Read the model definition and answer for the solid it produces. Units are mm, in the model's axes. Round coordinates to 2 decimals unless told otherwise and drop trailing zeros. Order: outer loops, then holes, each group sorted by start corner. A loop starts at its lowest first (then second) coordinate and runs counter-clockwise, first axis right, second up. Notation, with made-up numbers: (17, 48) - (55, 48) arc R23 cw to (55, 78) - close; hole circle Ø8 at (85, -7). An arc over 180 degrees is marked (long way). Answer as a JSON object with one key per item and string values. Group by question number.
Q1. A cutting plane is placed at C-C on x = -38. Determine the outline of the cut face in (y, z), and give its area (3 significant figures).
Q2. A cutting plane is placed at B-B on z = 0. Determine the outline of the cut face in (x, y).
Q3. A cutting plane is placed at D-D on y = -64.5. Determine the outline of the cut face in (x, z), and give its area (3 significant figures).
Q4. Given pin 1 Ø1 at (x, z) = (-33, 1) entering from +Y; pin 2 Ø2 at (y, z) = (-109.5, 0.5) entering from -X; pin 3 Ø1.2 at (y, z) = (-50.5, 0) entering from -X, each flat-ended and moving along its own axis, determine where each tip first touches the part or whether it passes through.
Q5. Consider line 1 (Z direction, x = -4, y = -113.5); line 2 (X direction, y = 2, z = 0.2); line 3 (X direction, y = -63.5, z = 1). Determine where each line is inside the solid, lowest interval first.
Q6. A cutting plane is placed at A-A on y = -10. Determine the outline of the cut face in (x, z), and give its area (3 significant figures).
```python
from build123d import *

# Parameters (mm, degrees)
PAD_DEPTH    = 2.4
POCKET_DEPTH = 1.2
CHAMFER_SIZE = 1


with BuildPart() as part:
    # Sketch001 → Pad (new body, symmetric)
    with BuildSketch(Plane.XY):
        with BuildLine():
            ThreePointArc((-35.969784, -57.54415), (-33.691358, -77.55321), (-29.473826, -97.244988))
            ThreePointArc((-29.473826, -97.244988), (-17.916413, -119.460908), (2, -134.64173))
            Line((2, -134.64173), (2, 84.534861))
            Line((-45.930419, 96.485256), (2, 84.534861))
            Line((-35.969784, -57.54415), (-45.930419, 96.485256))
        make_face()
    extrude(amount=PAD_DEPTH, both=True)

    # Sketch → Pocket (cut, symmetric)
    with BuildSketch(Plane.XY):
        with BuildLine():
            Line((0, 85.033517), (0, -130.966483))
            ThreePointArc((-27.154362, -96.628473), (-17.140793, -116.615568), (0, -130.966483))
            ThreePointArc((-33.574786, -57.389272), (-31.322854, -77.165669), (-27.154362, -96.628473))
            Line((-33.574786, -57.389272), (-43.485993, 95.875793))
            Line((-43.485993, 95.875793), (0, 85.033517))
        make_face()
    extrude(amount=POCKET_DEPTH, both=True, mode=Mode.SUBTRACT)

    # Chamfer
    chamfer_edges = [part.edges().sort_by_distance(p)[0] for p in [
        (2, -134.64173, 0),
    ]]
    chamfer(chamfer_edges, length=CHAMFER_SIZE)


solid = part.part
```
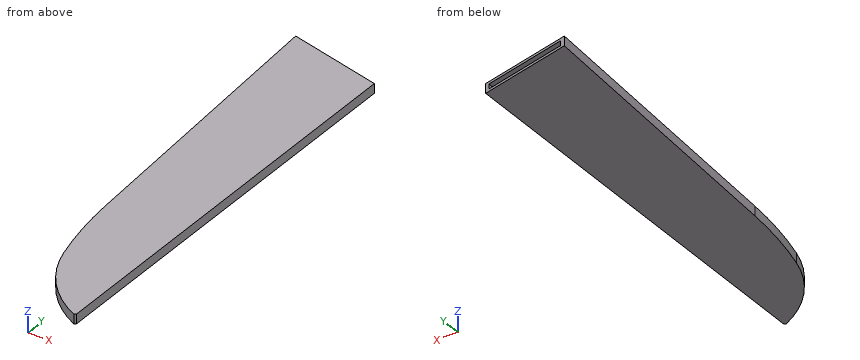
Result set:
{
 "1": {"outline": "(-26.15, -2.4) - (94.51, -2.4) - (94.51, -1.2) - (11.04, -1.2) - (11.04, 1.2) - (94.51, 1.2) - (94.51, 2.4) - (-26.15, 2.4) - close", "area": "379 mm²"},
 "2": {"outline": "(-45.93, 96.49) - (-35.97, -57.54) arc R206.4 ccw to (-29.47, -97.24) arc R57.4 ccw to (1.1, -134.22) - (2, -133.64) - (2, 84.53) - (0, 85.03) - (0, -130.97) arc R55 cw to (-27.15, -96.63) arc R204 cw to (-33.57, -57.39) - (-43.49, 95.88) - close"},
 "3": {"outline": "(-35.4, -2.4) - (2, -2.4) - (2, 2.4) - (-35.4, 2.4) - close; hole (-32.99, -1.2) - (0, -1.2) - (0, 1.2) - (-32.99, 1.2) - close", "area": "100 mm²"},
 "4": {"pin 1": "stops at y = 93.38", "pin 2": "stops at x = -25.17", "pin 3": "stops at x = -36.46"},
 "5": {"line 1": "z = -2.4 to -1.2, 1.2 to 2.4", "line 2": "x = -39.82 to -37.42, 0 to 2", "line 3": "x = -35.5 to -33.09, 0 to 2"},
 "6": {"outline": "(-39.04, -2.4) - (2, -2.4) - (2, 2.4) - (-39.04, 2.4) - close; hole (-36.64, -1.2) - (0, -1.2) - (0, 1.2) - (-36.64, 1.2) - close", "area": "109 mm²"}
}
